```python
from build123d import *

# Parameters (mm, degrees)
F0_W     = 6.35
F0_H     = 22.225
F1_DEPTH = 6.35
F2_W     = 4.7625
F2_H     = 20.6375
F3_DEPTH = 1.5875
F4_R     = 1.35255
F5_DEPTH = 6.35
F6_SIZE  = 3.57124


with BuildPart() as f1:
    # F0 (on Top) → F1 (new body)
    with BuildSketch(Plane.XY):
        with Locations((3.175, -11.1125)):
            Rectangle(F0_W, F0_H)
    extrude(amount=F1_DEPTH)

    # F2 (on face) → F3 (join)
    with BuildSketch(Plane.XY.offset(6.35)):
        with Locations((2.38125, -10.31875)):
            Rectangle(F2_W, F2_H)
    extrude(amount=F3_DEPTH)

    # F4 (on face) → F5 (cut)
    with BuildSketch(Plane(origin=(0, 0, 0), x_dir=(0, -1, 0), z_dir=(-1, 0, 0))):
        with Locations((17.4625, 3.175)):
            Circle(F4_R)
        with Locations((3.175, 3.175)):
            Circle(F4_R)
    extrude(amount=-F5_DEPTH, mode=Mode.SUBTRACT)

    # F6
    f6_edges = [f1.edges().sort_by_distance(p)[0] for p in [
        (4.7625, -20.6375, 7.14375),
    ]]
    chamfer(f6_edges, length=F6_SIZE)


solid = f1.part
```
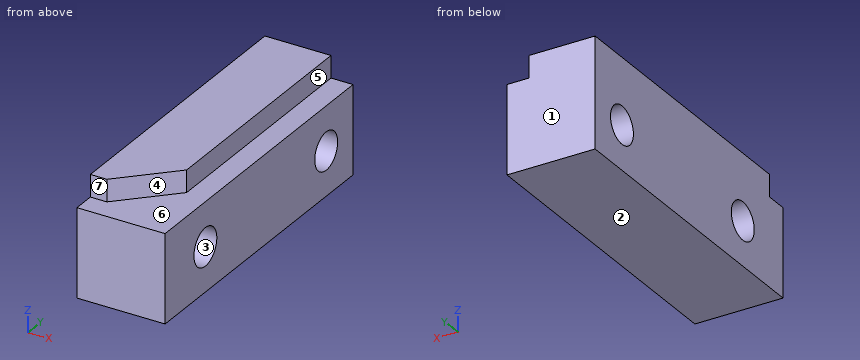
Model file for the job. Use its own axes, mm. Face numbers are marked on the shaded views. A direction names the side the tool comes from. Coordinates: 2 decimals unless noted, no trailing zeros. Loops run counter-clockwise (first coordinate to the right, second up) from the corner with the lowest first, then second, coordinate; pieces in that order, holes last. Notation, with made-up numbers: (-17.5, 68) - (-9.5, 68) arc R22 cw to (-9.5, 101) - close; hole circle Ø5 at (-19, -21.75). An arc over 180 degrees is marked (long way). Write item = value, one per line. Start each with the question number.
Item 1: Wall check: probe 1 along Y at (x, z) = (5.75, 4) (3 decimals); probe 2 along X at (y, z) = (-16.75, 6.5); probe 3 along Z at (x, y) = (5.5, -10.5). Give the ranges that are in metal, low to high. Write a range as [from, to].
Item 2: Saw through at B-B, the plane y = -4.25. List the corners of the cut face in (x, z).
Item 3: Saw through at A-A, the plane x = 3.5. State how many separate pieces and enclosed holes the cut face has, then the cut area to 3 significant figures.
Item 4: 3-axis set-ups, long thin cutter, end or side, ignore diameter. For the marked faces 5, 6 and 7: which of +Z, -Z, +X, -X, +Y, -Y reach the whole face in a straight line?
Item 5: Pull direction Y, two halves, no side cores. Call the marked faces 1, 2, 3 and 4: +Y half, -Y half, draft (parallel to the pull), parting line (faces both ways), or undercut.
Item 6: Saw through at C-C, the plane z = 4.25. List the corners of the cut face in (x, y) (3 decimals), then the cut area to 3 significant figures.
Answers:
q1.probe_1 = [-22.225, -18.534], [-16.391, -4.247], [-2.103, 0]
q1.probe_2 = [0, 4.76]
q1.probe_3 = [0, 6.35]
q2.outline = (0, 0) - (6.35, 0) - (6.35, 2.35) - (0, 2.35) - close; (0, 4) - (6.35, 4) - (6.35, 6.35) - (4.76, 6.35) - (4.76, 7.94) - (0, 7.94) - close
q3.separate_pieces = 1
q3.enclosed_holes = 2
q3.area = 159 mm2
q4.face_5 = +Z, +X, +Y, -Y
q4.face_6 = +Z, +X, -Y
q4.face_7 = +Z, +X, -X, -Y
q5.face_1 = +Y half
q5.face_2 = draft
q5.face_3 = undercut
q5.face_4 = -Y half
q6.outline = (0, -22.225) - (6.35, -22.225) - (6.35, -18.283) - (0, -18.283) - close; (0, -16.642) - (6.35, -16.642) - (6.35, -3.996) - (0, -3.996) - close; (0, -2.354) - (6.35, -2.354) - (6.35, 0) - (0, 0) - close
q6.area = 120 mm2
